For this review, take the finished solid that the model builds, in its own axes (mm). Face numbers are marked on the shaded views. A direction names the side the tool comes from. Give positions to 0.01 mm unless a question says otherwise; leave off trailing zeros. Write each loop counter-clockwise with the first axis right and the second up, starting at its lowest first coordinate (ties: lowest second). Pieces come first, ordered by that corner, then holes. Notation, with made-up numbers: (12, -24) -> (56, -24) arc R15 ccw to (56, -14) -> close; hole circle Ø3 at (62.5, 23). An arc over 180 degrees is marked (long way). Return JSON: item names as keys, results as strings.
from build123d import *

# Parameters (mm, degrees)
F1_R     = 10
F2_DEPTH = 7
F0_R     = 13
F3_DEPTH = 3


# Not quite as in the source:
# - a fillet or chamfer that OpenCascade refuses, or shapes differently, is made with other operations: its cross-section is extruded or revolved along the edge and cut away or added


with BuildPart() as f2:
    # F1 (on Top) → F2 (new body)
    with BuildSketch(Plane.XY):
        Circle(F1_R)
    extrude(amount=F2_DEPTH)

    # F0 (on Top) → F3 (join)
    with BuildSketch(Plane.XY):
        Circle(F0_R)
    extrude(amount=F3_DEPTH)

    # F4: fillet of radius 5 on 1 edges, made by hand

    # F4_s1 → F4_t2 (revolve, cut)
    with BuildSketch(Plane.XZ):
        with BuildLine():
            ThreePointArc((8.417424305, 0), (11.1560370926, 0.8166998673), (13, 3))
            Line((13, 3), (13, 0))
            Line((13, 0), (8.417424305, 0))
        make_face()
    revolve(axis=Axis((0, 0, 0), (0, 0, 1)), mode=Mode.SUBTRACT)


solid = f2.part
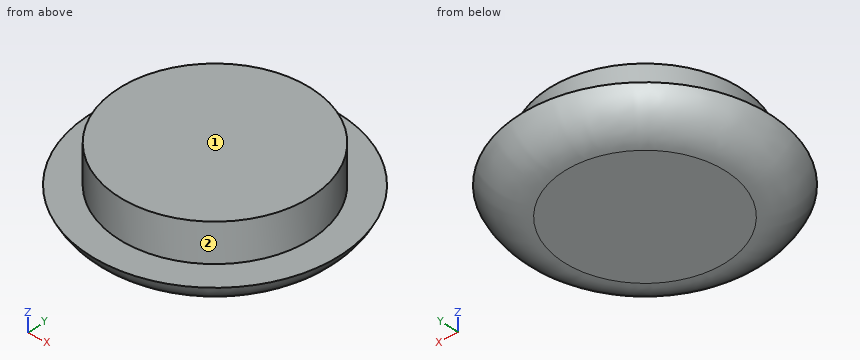
1. Add section C-C, the plane z = 5.5. State the section outline as (x, y) points.
Results found:
{"outline": "circle Ø20 at (0, 0)"}
2. Add section D-D, the plane z = 1. State the section outline as (x, y) points, plus the area to 3 significant figures.
Results found:
{"outline": "circle Ø22.83 at (0, 0)", "area": "410 mm²"}
3. Add section A-A, the plane x = 0. State the section outline as (y, z) points, plus the area to 3 significant figures.
Results found:
{"outline": "(-13, 3) arc R5 ccw to (-8.42, 0) -> (8.42, 0) arc R5 ccw to (13, 3) -> (10, 3) -> (10, 7) -> (-10, 7) -> (-10, 3) -> close", "area": "150 mm²"}
4. For pin 1 (4 mm diameter, centred on x = -0.5, z = 2.5, fed in from +Y); pin 2 (1 mm diameter, centred on y = -10, z = 1.5, fed in from +X), all flat-tipped, find the tip position at first contact; note any pin that passes through.
Results found:
{"pin 1": "stops at y = 13", "pin 2": "stops at x = 7.64"}
5. For the marked faces 1 and 2, list the 3-axis set-ups (+Z, -Z, +X, -X, +Y, -Y) from which the entire face can be reached by the end or side of a thin tool; tool diameter is ignored.
Results found:
{"face 1": "+Z, +X, -X, +Y, -Y", "face 2": "+Z"}
6. To check wall thickness, follow probe 1 along Y at (x, z) = (-6.75, 4.25); probe 2 along X at (y, z) = (-5.5, 6.75); probe 3 along X at (y, z) = (2.25, 5.5). State the ranges of each line that lie inside material, in increasing order.
Results found:
{"probe 1": "y = -7.38 to 7.38", "probe 2": "x = -8.35 to 8.35", "probe 3": "x = -9.74 to 9.74"}
